Geometry: final body of the model. Coordinates: model frame, mm. Face numbers are marked on the shaded views. A direction names the side the tool comes from. Give positions to 0.01 mm unless a question says otherwise; leave off trailing zeros. Loops run counter-clockwise (first coordinate to the right, second up) from the corner with the lowest first, then second, coordinate; pieces in that order, holes last. Notation, with made-up numbers: (17.25, 79) - (65.25, 79) arc R10 ccw to (65.25, 84) - close; hole circle Ø8 at (71.25, -8). An arc over 180 degrees is marked (long way). Answer in a Markdown table with one row per item.
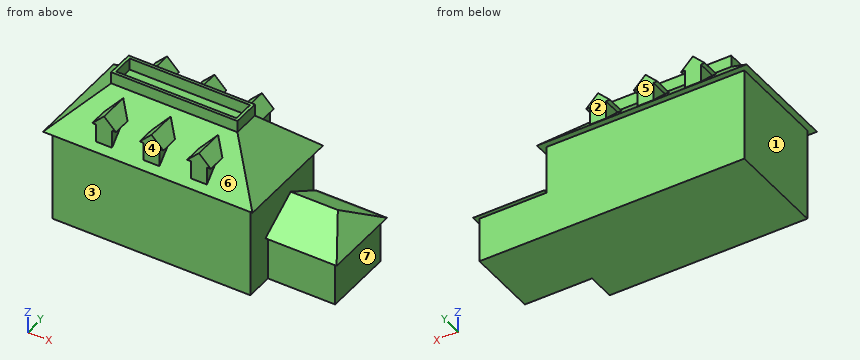
from build123d import *

# Parameters (mm, degrees)
F1_DEPTH       = 11.42979
F3_DEPTH       = 12.28684
F4_W           = 53
F4_H           = 28
F5_DEPTH       = 10.53635
F5_TAPER       = 45
F10_DEPTH      = 18
F12_DEPTH      = 19.501
F12_DEPTH_BACK = 8.501
F13_W          = 31.9273
F13_H          = 6.9273
F13_W_2        = 30.4412200116
F13_H_2        = 5.4412200116
F14_DEPTH      = 3


with BuildPart() as f1:
    # F0 (on Top) → F1 (new body)
    with BuildSketch(Plane.XY):
        Polygon((-25, -12.5), (25, -12.5), (25, -5.5), (42, -5.5), (42, 12.5), (25, 12.5), (-25, 12.5), align=None)
    extrude(amount=F1_DEPTH)

    # F2 (on face) → F3 (join)
    with BuildSketch(Plane.XY.offset(11.42979)):
        Polygon((-25, -12.5), (25, -12.5), (25, -5.5), (25, 12.5), (-25, 12.5), align=None)
    extrude(amount=F3_DEPTH)

    # F4 (on face) → F5 (join)
    with BuildSketch(Plane.XY.offset(23.71663)):
        Rectangle(F4_W, F4_H)
    extrude(amount=F5_DEPTH, taper=F5_TAPER)


with BuildPart() as f7:
    # F6 (on face) → F7 (new body, up to the next surface of F1)
    with BuildSketch(Plane.XZ.offset(12.5)):
        Polygon((-12, 32.8224519938), (-15, 29.8224519938), (-14, 29.8224519938), (-14, 25.21663), (-12, 25.21663), (-10, 25.21663), (-10, 29.8224519938), (-9, 29.8224519938), align=None)
    extrude(until=Until.NEXT, target=f1.part, dir=(0, 1, 0))


with BuildPart() as f7b:
    # F6 (on face) → F7, piece 2 (new body, up to the next surface of F1)
    with BuildSketch(Plane.XZ.offset(12.5)):
        Polygon((-2, 25.21663), (0, 25.21663), (2, 25.21663), (2, 29.8224519938), (3, 29.8224519938), (0, 32.8224519938), (-3, 29.8224519938), (-2, 29.8224519938), align=None)
    extrude(until=Until.NEXT, target=f1.part, dir=(0, 1, 0))


with BuildPart() as f7c:
    # F6 (on face) → F7, piece 3 (new body, up to the next surface of F1)
    with BuildSketch(Plane.XZ.offset(12.5)):
        Polygon((10, 25.21663), (12, 25.21663), (14, 25.21663), (14, 29.8224519938), (15, 29.8224519938), (12, 32.8224519938), (9, 29.8224519938), (10, 29.8224519938), align=None)
    extrude(until=Until.NEXT, target=f1.part, dir=(0, 1, 0))


with BuildPart() as f1_1:
    add(f1.part)

    # F8: F7, F7b, F7c across plane
    add(f7.part.mirror(Plane.XZ))
    add(f7b.part.mirror(Plane.XZ))
    add(f7c.part.mirror(Plane.XZ))

    # F9 (on face) → F10 (join)
    with BuildSketch(Plane.YZ.offset(25)):
        Polygon((3.5, 17.4922389561), (-6.5, 11.42979), (-5.5, 11.42979), (12.5, 11.42979), (12.5, 12.0360348956), align=None)
        Polygon((12.5, 12.0360348956), (12.5, 11.42979), (13.5, 11.42979), align=None)
    extrude(amount=F10_DEPTH)

    # F11 (on face) → F12 (cut, two sides)
    with BuildSketch(Plane.XZ.offset(5.5)) as f12_sk:
        Polygon((43, 11.42979), (43, 17.4922389561), (36.9375510439, 17.4922389561), align=None)
    extrude(amount=-F12_DEPTH, mode=Mode.SUBTRACT)
    extrude(f12_sk.sketch, amount=F12_DEPTH_BACK, mode=Mode.SUBTRACT)

    add(f7.part)  # F14 merges F7

    add(f7b.part)  # F14 merges F7b

    add(f7c.part)  # F14 merges F7c
    # F13 (on face) → F14 (join)
    with BuildSketch(Plane.XY.offset(34.25298)):
        Rectangle(F13_W, F13_H)
        Rectangle(F13_W_2, F13_H_2, mode=Mode.SUBTRACT)
    extrude(amount=F14_DEPTH)


solid = f1_1.part
Q1. First-contact query: pin 1 (2 mm diameter, centred on y = 10, z = 24.5, fed in from +X); pin 2 (5 mm diameter, centred on y = 9.5, z = 28, fed in from -X); pin 3 (5 mm diameter, centred on y = 9.5, z = 28, fed in from +X). Flat tips, straight axial feed; report the tip coordinate or a pass-through.
Check values:
| item | result |
|---|---|
| pin 1 | x = 26.5 |
| pin 2 | x = -24.72 |
| pin 3 | x = 24.72 |
Q2. Cut plane A-A (z = 8). Output: boundary loops of the cut face in (x, y), and give its area (3 significant figures).
Check values:
| item | result |
|---|---|
| outline | (-25, -12.5) - (25, -12.5) - (25, -5.5) - (42, -5.5) - (42, 12.5) - (-25, 12.5) - close |
| area | 1,560 mm² |
Q3. Draft query along X for the marked faces 5, 6 and 7. Return one class per face: pulls with the +X half, pulls with the -X half, needs draft (parallel to the pull), parting line crosses it, or undercut.
Check values:
| item | result |
|---|---|
| face 5 | needs draft |
| face 6 | undercut |
| face 7 | pulls with the +X half |
Q4. Cut plane B-B (x = -20). Output: boundary loops of the cut face in (y, z), and give its area (3 significant figures).
Check values:
| item | result |
|---|---|
| outline | (-14, 23.72) - (-12.5, 23.72) - (-12.5, 0) - (12.5, 0) - (12.5, 23.72) - (14, 23.72) - (7.5, 30.22) - (-7.5, 30.22) - close |
| area | 733 mm² |
Q5. Material intervals for line 1 along X through (y, z) = (11.5, 26.5); line 2 along X through (y, z) = (11.5, 3.5); line 3 along Z through (x, y) = (13.5, -2.25), sorted ascending.
Check values:
| item | result |
|---|---|
| line 1 | -14 to -10, -2 to 2, 10 to 14 |
| line 2 | -25 to 42 |
| line 3 | 0 to 34.25 |
Q6. Cut plane D-D (x = 29). Output: boundary loops of the cut face in (y, z).
Check values:
| item | result |
|---|---|
| outline | (-6.5, 11.43) - (-5.5, 11.43) - (-5.5, 0) - (12.5, 0) - (12.5, 11.43) - (13.5, 11.43) - (3.5, 17.49) - close |
Q7. Reachability of the marked faces 1, 2, 3 and 4 from +Z, -Z, +X, -X, +Y, -Y: full face, straight path, thin tool, end or side. Return the list, or none.
Check values:
| item | result |
|---|---|
| face 1 | -Z, -X, +Y, -Y |
| face 2 | +Z, +X, -X, +Y |
| face 3 | -Z, +X, -X, -Y |
| face 4 | +Z, +X, -X, -Y |
